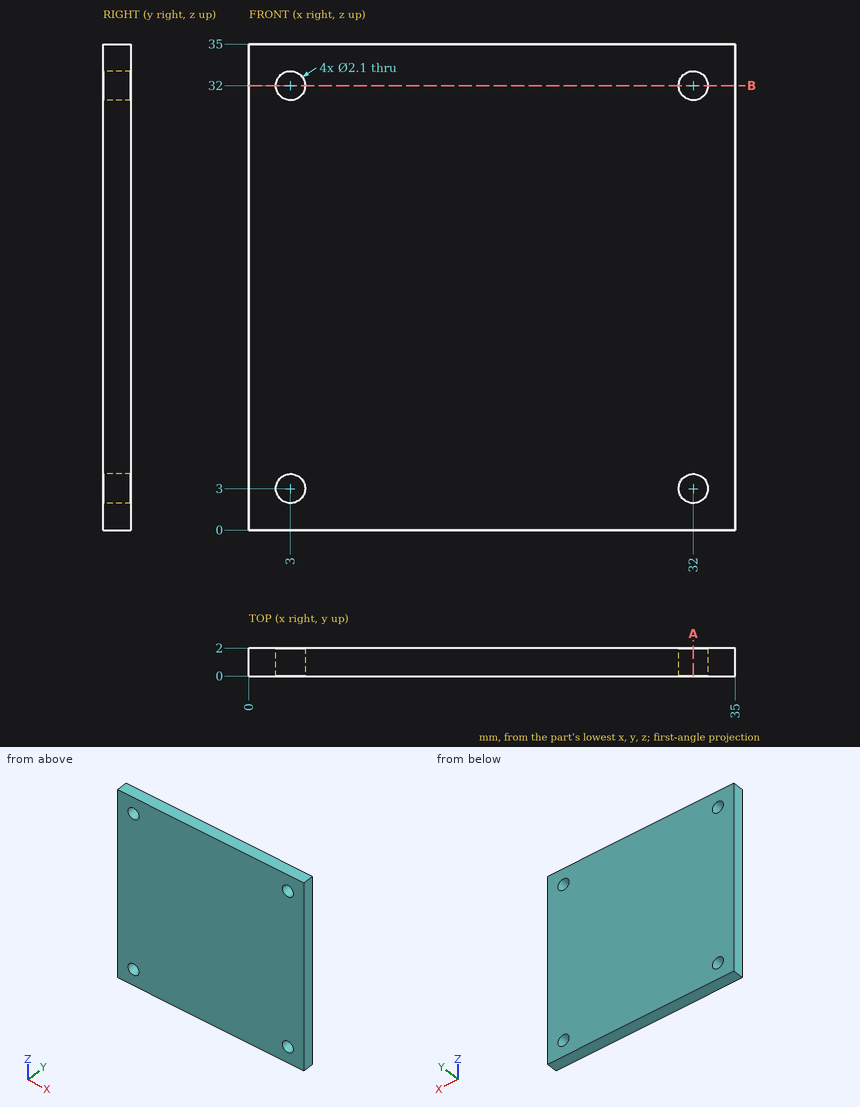
Study the drawing (mm; zero at the part's minimum x, y, z) and answer. Coordinates: 2 decimals unless noted, no trailing zeros. Write each loop counter-clockwise with the first axis right and the second up, starting at its lowest first coordinate (ties: lowest second). Pieces come first, ordered by that corner, then holes. Notation, with made-up numbers: (21, 55.5) - (62, 55.5) arc R16 ccw to (62, 66.5) - close; hole circle Ø3 at (81, -38). An arc over 180 degrees is marked (long way). Return JSON: item names as keys, results as strings. Group by question number.
1. A cutting plane is placed at B-B, the plane z = 32. Determine the outline of the cut face in (x, y).
2. Given pin 1 (1.9 mm diameter, centred on x = 3, z = 3, fed in from +Y) (1 decimal), flat-ended and moving along its own axis, determine where the tip first touches the part or whether it passes through.
3. A cutting plane is placed at A-A, the plane x = 32. Determine the outline of the cut face in (y, z).
4. Straight lines are drawn through the part: L1, parallel to Z at x = 3, y = 1.65; L2, parallel to Z at x = 3.5, y = 0.75. For each, find the intervals that lie inside material, in ascending order.
Ans:
{
 "1": {"outline": "(0, 0) - (1.95, 0) - (1.95, 2) - (0, 2) - close; (4.05, 0) - (30.95, 0) - (30.95, 2) - (4.05, 2) - close; (33.05, 0) - (35, 0) - (35, 2) - (33.05, 2) - close"},
 "2": {"pin 1": "through"},
 "3": {"outline": "(0, 0) - (2, 0) - (2, 1.95) - (0, 1.95) - close; (0, 4.05) - (2, 4.05) - (2, 30.95) - (0, 30.95) - close; (0, 33.05) - (2, 33.05) - (2, 35) - (0, 35) - close"},
 "4": {"L1": "0 to 1.95, 4.05 to 30.95, 33.05 to 35", "L2": "0 to 2.08, 3.92 to 31.08, 32.92 to 35"}
}
